from build123d import *

# Parameters (mm, degrees)
BOSS_EXTRUDE1_DEPTH      = 3
BOSS_EXTRUDE2_DEPTH      = 6
BOSS_EXTRUDE3_DEPTH      = 9.69
BOSS_EXTRUDE3_DEPTH_BACK = 6
FILLET1_R                = 2
FILLET2_R                = 2
BOSS_EXTRUDE4_DEPTH      = 40.233333333
CUT_EXTRUDE1_DEPTH       = 1.5
CUT_EXTRUDE2_DEPTH       = 1.5
BOSS_EXTRUDE5_DEPTH      = 54.58
CUT_EXTRUDE3_DEPTH       = 214.009386465
CUT_EXTRUDE3_DEPTH_BACK  = 214.009386465
SKETCH10_R               = 3.5
SKETCH12_W               = 12
SKETCH12_H               = 30.726270376
SKETCH12_W_2             = 4.828508562
SKETCH12_H_2             = 30.231621193
CUT_EXTRUDE4_DEPTH       = 5
SKETCH13_W               = 135.857143104
SKETCH13_H               = 55.923333333
BOSS_EXTRUDE6_DEPTH      = 1


with BuildPart() as part:
    # Sketch2 → Boss-Extrude1 (new body)
    with BuildSketch(Plane(origin=(0, 0, 0), x_dir=(1, 0, 0), z_dir=(0, 1, 0))):
        with BuildLine():
            Line((-44.358814779, -15.844661539), (100.530059165, -54.667518304))
            Line((100.530059165, -54.667518304), (100.530059165, 51.906312945))
            Line((100.530059165, 51.906312945), (-44.358814779, 13.083456179))
            ThreePointArc((-44.358814779, 13.083456179), (-53.518419956, -1.38060268), (-44.358814779, -15.844661539))
        make_face()
    extrude(amount=BOSS_EXTRUDE1_DEPTH)

    # Sketch2<3> → Boss-Extrude2 (add)
    with BuildSketch(Plane(origin=(0, 0, 0), x_dir=(1, 0, 0), z_dir=(0, 1, 0))):
        with BuildLine():
            Line((-44.358814779, 13.083456179), (100.530059165, 51.906312945))
            Line((100.530059165, 51.906312945), (100.530059165, -54.667518304))
            Line((100.530059165, -54.667518304), (-44.358814779, -15.844661539))
            ThreePointArc((-44.358814779, -15.844661539), (-53.518419956, -1.38060268), (-44.358814779, 13.083456179))
        make_face()
        with BuildLine():
            Line((-46.067020476, 4.994507774), (35.007341865, 26.71831769))
            ThreePointArc((35.007341865, 26.71831769), (38.656739262, -1.38060268), (35.007341865, -29.479523049))
            Line((35.007341865, -29.479523049), (-46.067020476, -7.755713133))
            ThreePointArc((-46.067020476, -7.755713133), (-51.145215007, -1.38060268), (-46.067020476, 4.994507774))
        make_face(mode=Mode.SUBTRACT)
    extrude(amount=BOSS_EXTRUDE2_DEPTH)

    # Sketch3 → Boss-Extrude3 (add, two sides: drawn at the far end of the back side and taken through both)
    with BuildSketch(Plane(origin=(0, 6, 0), x_dir=(1, 0, 0), z_dir=(0, 1, 0)).offset(-BOSS_EXTRUDE3_DEPTH_BACK)):
        with BuildLine():
            Line((44.072517202, -66.967163029), (44.072517202, -39.539765529))
            Line((44.072517202, -39.539765529), (44.072517202, 36.778560169))
            Line((44.072517202, 36.778560169), (44.072517202, 63.981792798))
            ThreePointArc((44.072517202, 63.981792798), (44.650972897, 65.388637419), (46.051728991, 65.981684758))
            Line((46.051728991, 65.981684758), (100.530059165, 66.547968872))
            Line((100.530059165, 66.547968872), (100.530059165, 51.906312945))
            Line((100.530059165, 51.906312945), (100.530059165, -54.667518304))
            Line((100.530059165, -54.667518304), (100.530059165, -69.309174232))
            Line((100.530059165, -69.309174232), (46.059958243, -68.967123596))
            ThreePointArc((46.059958243, -68.967123596), (44.653870326, -68.376929336), (44.072517202, -66.967163029))
        make_face()
    extrude(amount=BOSS_EXTRUDE3_DEPTH + BOSS_EXTRUDE3_DEPTH_BACK)

    # Fillet1
    fillet1_edges = [part.edges().sort_by_distance(p)[0] for p in [
        (44.072517202, 3, 39.539765529),
    ]]
    fillet(fillet1_edges, radius=FILLET1_R)

    # Fillet2
    fillet2_edges = [part.edges().sort_by_distance(p)[0] for p in [
        (44.072517202, 3, -36.778560169),
    ]]
    fillet(fillet2_edges, radius=FILLET2_R)

    # Sketch5 → Boss-Extrude4 (add)
    with BuildSketch(Plane(origin=(0, 15.69, 0), x_dir=(1, 0, 0), z_dir=(0, 1, 0))):
        with BuildLine():
            Line((46.059958243, -68.967123596), (100.530059165, -69.309174232))
            Line((100.530059165, -69.309174232), (100.530059165, 66.547968872))
            Line((100.530059165, 66.547968872), (46.051728991, 65.981684758))
            ThreePointArc((46.051728991, 65.981684758), (44.650972897, 65.388637419), (44.072517202, 63.981792798))
            Line((44.072517202, 63.981792798), (44.072517202, -66.967163029))
            ThreePointArc((44.072517202, -66.967163029), (44.653870326, -68.376929336), (46.059958243, -68.967123596))
        make_face()
        with BuildLine():
            Line((99.530059165, -68.302874912), (99.530059165, 65.537520182))
            Line((99.530059165, 65.537520182), (46.062123097, 64.981738778))
            ThreePointArc((46.062123097, 64.981738778), (45.36174505, 64.685215109), (45.072517202, 63.981792798))
            Line((45.072517202, 63.981792798), (45.072517202, -66.967163029))
            ThreePointArc((45.072517202, -66.967163029), (45.363193764, -67.672046182), (46.066237723, -67.967143312))
            Line((46.066237723, -67.967143312), (99.530059165, -68.302874912))
        make_face(mode=Mode.SUBTRACT)
    extrude(amount=BOSS_EXTRUDE4_DEPTH)

    # Sketch6 → Cut-Extrude1 (cut)
    with BuildSketch(Plane.ZY.offset(-44.072517202)):
        with BuildLine():
            add(Edge.make_bspline(
                [(-15.745078449, 23.050825441), (-16.426574269, 23.424993836), (-18.107694271, 23.59390395), (-20.06054673, 21.997763181), (-20.359072413, 19.493331011), (-18.791777494, 17.501685815), (-16.270097491, 17.248320643), (-14.317245033, 18.844461412), (-14.018719349, 21.348893583), (-15.063582628, 22.676657046), (-15.745078449, 23.050825441)],
                knots=[0, 0, 0, 0, 0.785398163, 1.570796327, 2.35619449, 3.141592654, 3.926990817, 4.71238898, 5.497787144, 6.283185307, 6.283185307, 6.283185307, 6.283185307], degree=3))
        make_face()
        with BuildLine():
            add(Edge.make_bspline(
                [(4.422895342, 20.879911755), (4.30327296, 21.652897904), (3.419826029, 23.099177602), (0.951461151, 23.695508582), (-1.221188854, 22.380963882), (-1.828624955, 19.912466539), (-0.50345456, 17.743046992), (1.964910319, 17.146716012), (4.137560324, 18.461260712), (4.542517725, 20.106925607), (4.422895342, 20.879911755)],
                knots=[0, 0, 0, 0, 0.785398163, 1.570796327, 2.35619449, 3.141592654, 3.926990817, 4.71238898, 5.497787144, 6.283185307, 6.283185307, 6.283185307, 6.283185307], degree=3))
        make_face()
        with BuildLine():
            add(Edge.make_bspline(
                [(20.102815045, 23.421112297), (19.325002738, 23.421112297), (17.769378124, 22.760793636), (16.823992487, 20.421112297), (17.769378124, 18.081430957), (20.102815045, 17.090952967), (22.436251966, 18.081430957), (23.381637603, 20.421112297), (22.436251966, 22.760793636), (20.880627352, 23.421112297), (20.102815045, 23.421112297)],
                knots=[0, 0, 0, 0, 0.785398163, 1.570796327, 2.35619449, 3.141592654, 3.926990817, 4.71238898, 5.497787144, 6.283185307, 6.283185307, 6.283185307, 6.283185307], degree=3))
        make_face()
    extrude(amount=-CUT_EXTRUDE1_DEPTH, mode=Mode.SUBTRACT)

    # Sketch7 → Cut-Extrude2 (cut)
    with BuildSketch(Plane(origin=(100.530059165, 0, 0), x_dir=(0, 0, -1), z_dir=(1, 0, 0))):
        with BuildLine():
            Line((-51.487685115, 48.534557921), (-41.492685115, 48.534557921))
            ThreePointArc((-41.492685115, 48.534557921), (-39.98663504, 47.028507846), (-41.492685115, 45.522457772))
            Line((-41.492685115, 45.522457772), (-51.487685115, 45.522457772))
            ThreePointArc((-51.487685115, 45.522457772), (-52.99373519, 47.028507846), (-51.487685115, 48.534557921))
        make_face()
        with BuildLine():
            Line((-6.487685115, 48.534557921), (3.507314885, 48.534557921))
            ThreePointArc((3.507314885, 48.534557921), (5.013364959, 47.028507846), (3.507314885, 45.522457772))
            Line((3.507314885, 45.522457772), (-6.487685115, 45.522457772))
            ThreePointArc((-6.487685115, 45.522457772), (-7.99373519, 47.028507846), (-6.487685115, 48.534557921))
        make_face()
        with BuildLine():
            Line((38.512314885, 48.534557921), (48.507314885, 48.534557921))
            ThreePointArc((48.507314885, 48.534557921), (50.01336496, 47.028507846), (48.507314885, 45.522457772))
            Line((48.507314885, 45.522457772), (38.512314885, 45.522457772))
            ThreePointArc((38.512314885, 45.522457772), (37.00626481, 47.028507846), (38.512314885, 48.534557921))
        make_face()
    extrude(amount=-CUT_EXTRUDE2_DEPTH, mode=Mode.SUBTRACT)

    # Sketch8 → Boss-Extrude5 (add)
    with BuildSketch(Plane(origin=(100.530059165, 0, 0), x_dir=(0, 0, -1), z_dir=(1, 0, 0))):
        Polygon((66.547968872, 55.923333333), (66.547968872, 0), (-69.309174232, 0), (-69.309174232, 55.923333333), (-68.309174232, 55.923333333), (-68.309174232, 1), (65.547968872, 1), (65.547968872, 55.923333333), align=None)
    extrude(amount=BOSS_EXTRUDE5_DEPTH)

    # Sketch10 → Cut-Extrude3 (cut, two sides: drawn at the far end of the back side and taken through both)
    with BuildSketch(Plane.XY.offset(-65.547968872).offset(-CUT_EXTRUDE3_DEPTH_BACK)):
        with Locations((126.491326957, 23.246690768)):
            Circle(SKETCH10_R)
    extrude(amount=CUT_EXTRUDE3_DEPTH + CUT_EXTRUDE3_DEPTH_BACK, mode=Mode.SUBTRACT)

    # Sketch12 → Cut-Extrude4 (cut)
    with BuildSketch(Plane(origin=(0, 6, 0), x_dir=(1, 0, 0), z_dir=(0, 1, 0))):
        with Locations((13.982227259, -26.342654968)):
            Rectangle(SKETCH12_W, SKETCH12_H)
        with Locations((-20.920113411, -14.480437774)):
            Rectangle(SKETCH12_W_2, SKETCH12_H_2)
    extrude(amount=-CUT_EXTRUDE4_DEPTH, mode=Mode.SUBTRACT)

    # Sketch13 → Boss-Extrude6 (add)
    with BuildSketch(Plane(origin=(155.110059165, 0, 0), x_dir=(0, 0, -1), z_dir=(1, 0, 0))):
        with Locations((-1.38060268, 27.961666667)):
            Rectangle(SKETCH13_W, SKETCH13_H)
    extrude(amount=BOSS_EXTRUDE6_DEPTH)


solid = part.part
Source: CAD feature listing. Evaluate the final solid. Frame: model axes, mm. A direction names the side the tool comes from. Give positions to 0.01 mm unless a question says otherwise; leave off trailing zeros. Loops run counter-clockwise (first coordinate to the right, second up) from the corner with the lowest first, then second, coordinate; pieces in that order, holes last. Notation, with made-up numbers: (27.5, 69) -> (44.5, 69) arc R19 ccw to (44.5, 85) -> close; hole circle Ø11 at (-11.75, 85.25). An arc over 180 degrees is marked (long way). Use a Markdown table: item, result. Add a question column.
1) Pull-direction query (Z, two-part tool) for faces 1 (the face through (-18.506, 2, 14)), 2 (the face through (127, 29, 68.309)), 3 (the face through (-53.516, 2.958, 1.128)); classes: +Z half, -Z half, draft (parallel to the pull), parting line (faces both ways), or undercut.
2) First-contact query: pin 1 (4.5 mm diameter, centred on x = -10.5, z = 19.5, fed in from +Y); pin 2 (10 mm diameter, centred on x = 45, y = 7, fed in from +Z); pin 3 (2 mm diameter, centred on x = 12.5, y = 2.5, fed in from +Z); pin 4 (1.5 mm diameter, centred on x = -14, y = 7.5, fed in from -Z). Flat tips, straight axial feed; report the tip coordinate or a pass-through.
3) Section query D-D, the plane x = 22.5. Return the cut outline in (y, z), then the cut area to 3 significant figures.
4) Line query: line 1 along X through (y, z) = (37.5, -7.5); line 2 along Z through (x, y) = (116, 24.5); line 3 along Y through (x, z) = (84.5, 51.5). Output: solid intervals per line, ascending. Write a range as [from, to].
5) Section query A-A, the plane z = 45. Return the cut outline in (x, y), then the cut area to 3 significant figures.
6) Reachability of faces 4 (the face through (156.11, 28, 2)), 5 (the face through (-5, 6, 22)), 6 (the face through (7.982, 3, 23)), 7 (the face through (127, 28, -65.548)) from +Z, -Z, +X, -X, +Y, -Y: full face, straight path, thin tool, end or side. Return the list, or none.
7) Section query C-C, the plane z = -58. Return the cut outline in (x, y), then the cut area to 3 significant figures.
8) Section query B-B, the plane y = 29. Return the cut outline in (x, z).
Numbers:
| question | item | result |
|---|---|---|
| 1 | face 1 | draft |
| 1 | face 2 | undercut |
| 1 | face 3 | parting line |
| 2 | pin 1 | stops at y = 6 |
| 2 | pin 2 | stops at z = 68.99 |
| 2 | pin 3 | stops at z = 10.98 |
| 2 | pin 4 | passes through |
| 3 | outline | (0, -31) -> (6, -31) -> (6, -23.37) -> (3, -23.37) -> (3, 26.13) -> (6, 26.13) -> (6, 33.76) -> (0, 33.76) -> close |
| 3 | area | 240 mm2 |
| 4 | line 1 | x = [44.07, 45.07], [99.53, 100.53], [155.11, 156.11] |
| 4 | line 2 | z = [-66.55, -65.55], [68.31, 69.31] |
| 4 | line 3 | y = [0, 15.69] |
| 5 | outline | (44.07, 0) -> (156.11, 0) -> (156.11, 55.92) -> (155.11, 55.92) -> (155.11, 1) -> (100.53, 1) -> (100.53, 45.52) -> (99.53, 45.52) -> (99.53, 15.69) -> (45.07, 15.69) -> (45.07, 55.92) -> (44.07, 55.92) -> close; (99.53, 48.53) -> (100.53, 48.53) -> (100.53, 55.92) -> (99.53, 55.92) -> close |
| 5 | area | 1,070 mm2 |
| 6 | face 4 | +Z, -Z, +X, +Y, -Y |
| 6 | face 5 | +Z, -Z, -X, +Y |
| 6 | face 6 | +Z, +Y |
| 6 | face 7 | +Y |
| 7 | outline | (44.07, 0) -> (156.11, 0) -> (156.11, 55.92) -> (155.11, 55.92) -> (155.11, 1) -> (100.53, 1) -> (100.53, 55.92) -> (99.53, 55.92) -> (99.53, 15.69) -> (45.07, 15.69) -> (45.07, 55.92) -> (44.07, 55.92) -> close |
| 7 | area | 1,080 mm2 |
| 8 | outline | (44.07, -63.98) arc R2 ccw to (46.05, -65.98) -> (100.53, -66.55) -> (156.11, -66.55) -> (156.11, 69.31) -> (100.53, 69.31) -> (46.06, 68.97) arc R2 ccw to (44.07, 66.97) -> close; hole (45.07, -63.98) arc R1 ccw to (46.06, -64.98) -> (99.53, -65.54) -> (99.53, 68.3) -> (46.07, 67.97) arc R1 ccw to (45.07, 66.97) -> close; hole (100.53, -65.55) -> (155.11, -65.55) -> (155.11, 68.31) -> (100.53, 68.31) -> close |
